Check sheet for the drawn part. Datum: minimum x, y, z corner. Units: mm. A direction names the side the tool comes from. Give positions to 0.01 mm unless a question says otherwise; leave off trailing zeros. Order: outer loops, then holes, each group sorted by start corner. A loop starts at its lowest first (then second) coordinate and runs counter-clockwise, first axis right, second up. Notation, with made-up numbers: (70, 86.5) - (118, 86.5) arc R8 cw to (118, 96.5) - close; hole circle Ø5 at (-35.5, 48.5). An arc over 180 degrees is marked (long way). Answer as a JSON object with one key per item and string values. Group by question number.
(1) Section check D-D (x = 524). Record the boundary of the cut face in (y, z).
(2) Section check C-C (y = 478). Record the boundary of the cut face in (x, z), then the cut area to 4 significant figures.
(3) Section check B-B (z = 147). Record the boundary of the cut face in (x, y).
(4) Thickness scan on line 1 (X direction, y = 166, z = 25); line 2 (Y direction, x = 703, z = 158); line 3 (X direction, y = 520, z = 23.5). Record the ranges inside material, lowest first.
(5) Section check A-A (y = 165). Record the boundary of the cut face in (x, z).
(6) Access from +Z, -Z, +X, -X, +Y, -Y to the whole of each face (thin tool, end or side, straight path). Record for the marked faces 1 and 2.
(7) Depth check by flat-ended pin: pin 1 Ø17.5 at (y, z) = (238.5, 163.5) entering from -X; pin 2 Ø17.5 at (x, z) = (75.5, 10.5) entering from +Y; pin 3 Ø12 at (x, y) = (587, 324) entering from +Z. Enter the tip coordinate at first touch or a pass-through.
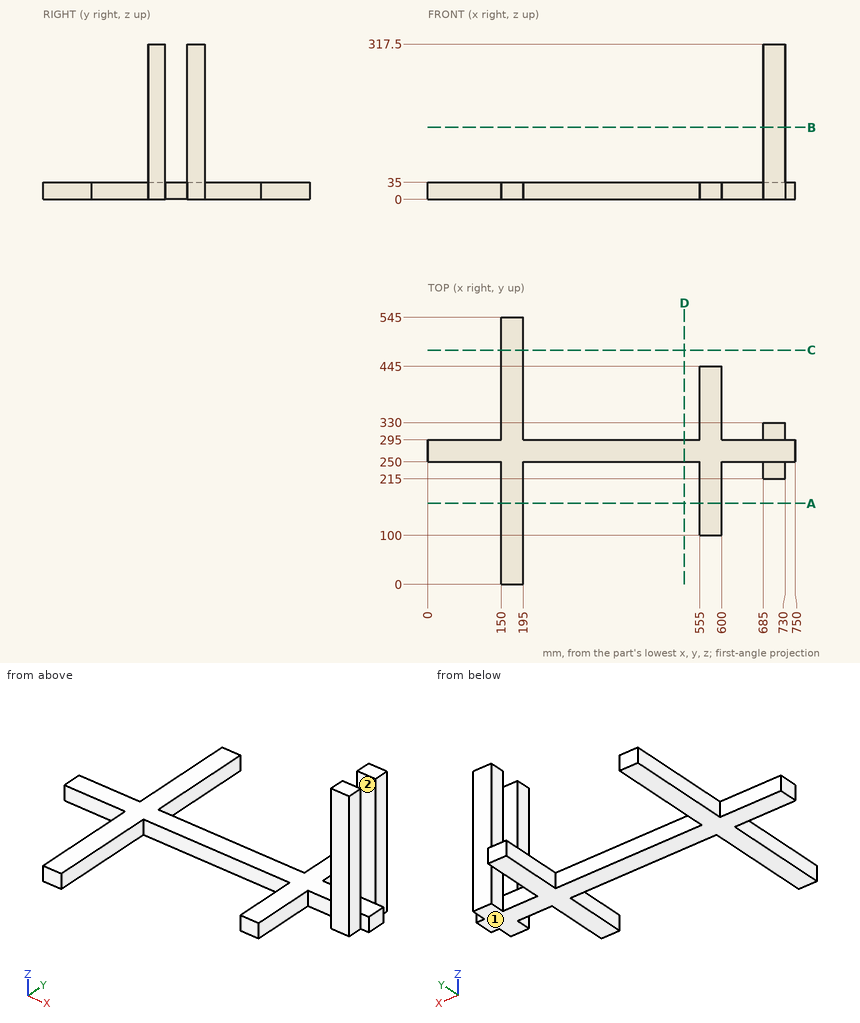
Solutions:
{
 "1": {"outline": "(250, 0) - (295, 0) - (295, 35) - (250, 35) - close"},
 "2": {"outline": "(150, 0) - (195, 0) - (195, 35) - (150, 35) - close", "area": "1,575 mm2"},
 "3": {"outline": "(685, 215) - (730, 215) - (730, 250) - (685, 250) - close; (685, 295) - (730, 295) - (730, 330) - (685, 330) - close"},
 "4": {"line 1": "x = 150 to 195, 555 to 600", "line 2": "y = 215 to 250, 295 to 330", "line 3": "x = 150 to 195"},
 "5": {"outline": "(150, 0) - (195, 0) - (195, 35) - (150, 35) - close; (555, 0) - (600, 0) - (600, 35) - (555, 35) - close"},
 "6": {"face 1": "-Z, +X, -X, +Y, -Y", "face 2": "+Z, +X, -X"},
 "7": {"pin 1": "stops at x = 685", "pin 2": "stops at y = 295", "pin 3": "stops at z = 35"}
}
